Could you check a few things on this drawing? It's one solid part, dimensions in mm from its lowest x, y, z. A direction names the side the tool comes from. Give positions to 0.01 mm unless a question says otherwise; leave off trailing zeros. Order: outer loops, then holes, each group sorted by start corner. A loop starts at its lowest first (then second) coordinate and runs counter-clockwise, first axis right, second up.
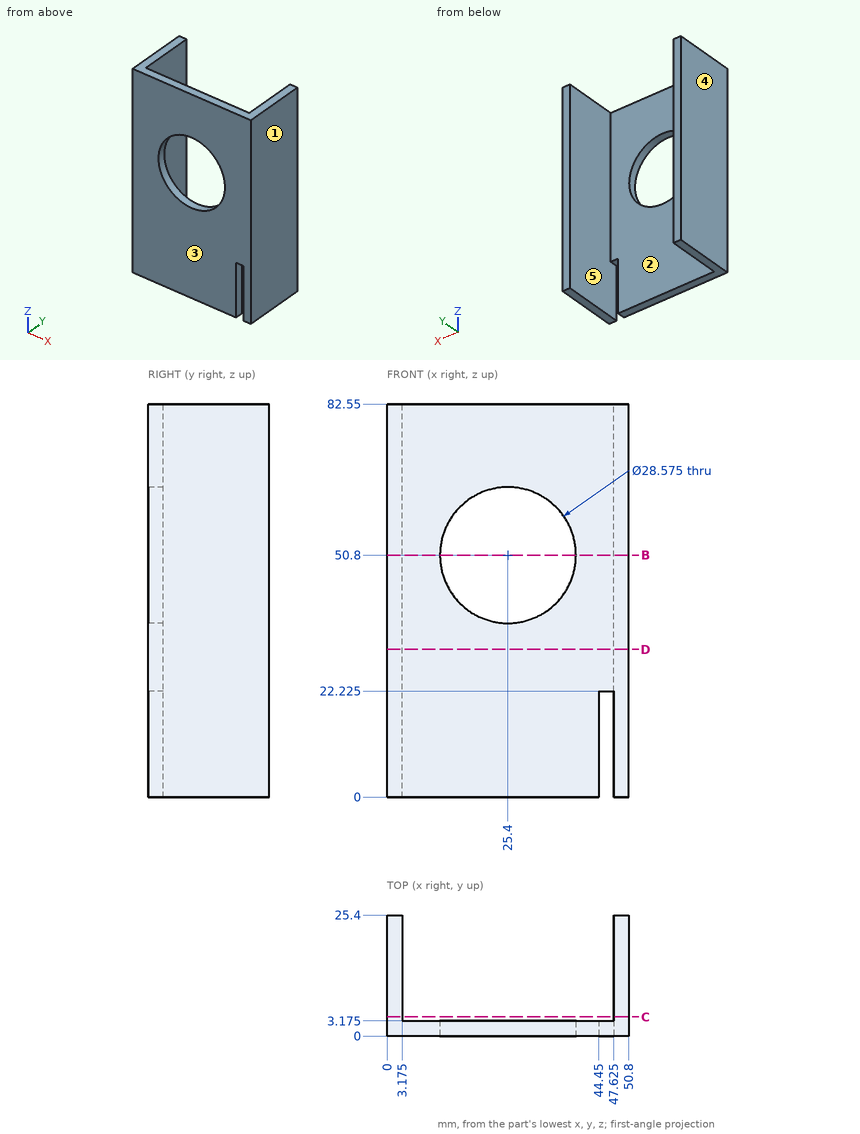
Item 1: For pin 1 (10 mm diameter, centred on x = 14, z = 67.5, fed in from +Y) (3 decimals); pin 2 (23 mm diameter, centred on x = 25.4, z = 50.8, fed in from +Y), each with a flat end and sliding along its axis, tell me the tip position at first contact or that it passes through.
Findings:
pin 1: stops at y = 3.175
pin 2: passes through
Item 2: Imagine slicing it at B-B on z = 50.8. List the corners of the cut face in (x, y) for me (1 decimal).
Findings:
outline: (0, 0) - (11.1, 0) - (11.1, 3.2) - (3.2, 3.2) - (3.2, 25.4) - (0, 25.4) - close; (39.7, 0) - (50.8, 0) - (50.8, 25.4) - (47.6, 25.4) - (47.6, 3.2) - (39.7, 3.2) - close
Item 3: Please list where these lines run through material, in increasing order: line 1 along X through (y, z) = (7.5, 5) (3 decimals); line 2 along Z through (x, y) = (25.4, 1.65); line 3 along Y through (x, z) = (39.5, 23) (3 decimals).
Findings:
line 1: x = 0 to 3.175, 47.625 to 50.8
line 2: z = 0 to 36.51, 65.09 to 82.55
line 3: y = 0 to 3.175
Item 4: For the marked faces 1 and 2, which set-ups out of +Z, -Z, +X, -X, +Y, -Y let a thin tool reach every point of the face, with its end or its side?
Findings:
face 1: +Z, -Z, +X, +Y, -Y
face 2: +Z, -Z, +Y
Item 5: Imagine slicing it at D-D on z = 31. List the corners of the cut face in (x, y) for me (3 decimals).
Findings:
outline: (0, 0) - (50.8, 0) - (50.8, 25.4) - (47.625, 25.4) - (47.625, 3.175) - (3.175, 3.175) - (3.175, 25.4) - (0, 25.4) - close
Item 6: We'd pull the mould along X, two halves only. Please class the marked faces 3, 4 and 5: +X half, -X half, draft (parallel to the pull), parting line (faces both ways), or undercut.
Findings:
face 3: draft
face 4: -X half
face 5: undercut
Item 7: Imagine slicing it at C-C on y = 4. List the corners of the cut face in (x, z) for me (3 decimals).
Findings:
outline: (0, 0) - (3.175, 0) - (3.175, 82.55) - (0, 82.55) - close; (47.625, 0) - (50.8, 0) - (50.8, 82.55) - (47.625, 82.55) - close
